from build123d import *

# Parameters (mm, degrees)
SKETCH2_R           = 1.4
BOSS_EXTRUDE1_DEPTH = 21
CHAMFER2_SIZE       = 0.05
SKETCH3_R           = 2
BOSS_EXTRUDE2_DEPTH = 1


with BuildPart() as part:
    # Sketch2 → Boss-Extrude1 (new body)
    with BuildSketch(Plane.XY):
        with Locations(Location((0, 0, 0), (0, 0, 180))):
            Circle(SKETCH2_R)
    extrude(amount=BOSS_EXTRUDE1_DEPTH)

    # Chamfer2
    chamfer2_edges = [part.edges().sort_by_distance(p)[0] for p in [
        (1.4, 0, 0),
        (1.4, 0, 21),
    ]]
    chamfer(chamfer2_edges, length=CHAMFER2_SIZE)

    # Sketch3 → Boss-Extrude2 (add)
    with BuildSketch(Plane.XY.offset(21)):
        Circle(SKETCH3_R)
    extrude(amount=BOSS_EXTRUDE2_DEPTH)


solid = part.part
Here's how the part is built. I have some questions about the finished solid (model axes, mm). A direction names the side the tool comes from. Coordinates: 2 decimals unless noted, no trailing zeros. Order: outer loops, then holes, each group sorted by start corner. A loop starts at its lowest first (then second) coordinate and runs counter-clockwise, first axis right, second up. Notation, with made-up numbers: (-11.5, 45.25) -> (32.5, 45.25) arc R24 cw to (32.5, 59.25) -> close; hole circle Ø8 at (-0.5, -11.5). An arc over 180 degrees is marked (long way). Answer in a Markdown table with one row per item.
(1) I want a section at D-D on x = 1.65. List the corners of the cut face in (y, z) for me, then the cut area to 3 significant figures.
Answer key:
| item | result |
|---|---|
| outline | (-1.13, 21) -> (1.13, 21) -> (1.13, 22) -> (-1.13, 22) -> close |
| area | 2.26 mm^2 |
(2) On a 3-axis mill with a long thin cutter (end or side, diameter ignored), from which of +Z, -Z, +X, -X, +Y, -Y can I reach the whole of each face in a straight line? I mean faces 1 (the face through (1.4, -0.06, 10.35)), 2 (the face through (0, 0, 22)). Say none if no direction works.
Answer key:
| item | result |
|---|---|
| face 1 | -Z |
| face 2 | +Z, +X, -X, +Y, -Y |
(3) I want a section at A-A on x = 0. List the corners of the cut face in (y, z) for me.
Answer key:
| item | result |
|---|---|
| outline | (-2, 21) -> (-1.35, 21) -> (-1.4, 20.95) -> (-1.4, 0.05) -> (-1.35, 0) -> (1.35, 0) -> (1.4, 0.05) -> (1.4, 20.95) -> (1.35, 21) -> (2, 21) -> (2, 22) -> (-2, 22) -> close |
(4) I want a section at C-C on z = 12.5. List the corners of the cut face in (x, y) for me.
Answer key:
| item | result |
|---|---|
| outline | circle Ø2.8 at (0, 0) |
(5) Please list where these lines run through material, in increasing order: probe 1 along X at (y, z) = (-0.1, 1.5); probe 2 along Y at (x, z) = (-0.35, 4.25); probe 3 along Z at (x, y) = (1.5, -0.25).
Answer key:
| item | result |
|---|---|
| probe 1 | -1.4 to 1.4 |
| probe 2 | -1.36 to 1.36 |
| probe 3 | 21 to 22 |
(6) Will these pins go through, and if not, where does the flat tip stop? pin 1 Ø1 at (x, z) = (0, 16) entering from +Y; pin 2 Ø2 at (x, z) = (1, 3.5) entering from -Y; pin 3 Ø1 at (y, z) = (-0.5, 17) entering from +X.
Answer key:
| item | result |
|---|---|
| pin 1 | y = 1.4 |
| pin 2 | y = -1.4 |
| pin 3 | x = 1.4 |
